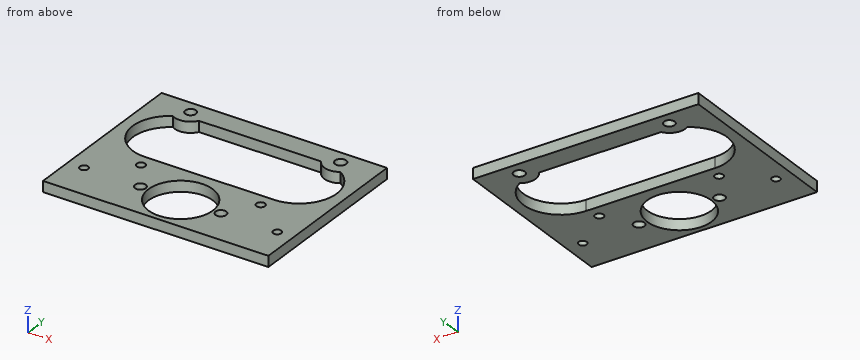
```python
from build123d import *

# Parameters (mm, degrees)
SKETCH1_W           = 133.35
SKETCH1_H           = 104.775
SKETCH1_R           = 2.413
SKETCH1_R_2         = 2.5273
SKETCH1_R_3         = 3.175
SKETCH1_R_4         = 19.05
SKETCH1_R_5         = 3.302
BOSS_EXTRUDE1_DEPTH = 6.35


with BuildPart() as part:
    # Sketch1 → Boss-Extrude1 (new body)
    with BuildSketch(Plane.XY):
        with Locations((0, 30.353)):
            Rectangle(SKETCH1_W, SKETCH1_H)
        with Locations((-57.15, 0)):
            Circle(SKETCH1_R, mode=Mode.SUBTRACT)
        with Locations((-35.41150672, 17.8308)):
            Circle(SKETCH1_R_2, mode=Mode.SUBTRACT)
        with Locations((-23.8125, 0)):
            Circle(SKETCH1_R_3, mode=Mode.SUBTRACT)
        Circle(SKETCH1_R_4, mode=Mode.SUBTRACT)
        with Locations((23.8125, 0)):
            Circle(SKETCH1_R_3, mode=Mode.SUBTRACT)
        with Locations((35.41150672, 17.8308)):
            Circle(SKETCH1_R_2, mode=Mode.SUBTRACT)
        with Locations((57.15, 0)):
            Circle(SKETCH1_R, mode=Mode.SUBTRACT)
        with Locations((44.64152658, 74.693330266)):
            Circle(SKETCH1_R_5, mode=Mode.SUBTRACT)
        with Locations((-44.258181609, 74.921110792)):
            Circle(SKETCH1_R_3, mode=Mode.SUBTRACT)
        with BuildLine():
            Line((-36.078617849, 70.0405), (36.185033541, 70.0405))
            ThreePointArc((36.185033541, 70.0405), (42.31521137, 65.325867347), (49.938818951, 66.624885711))
            ThreePointArc((49.938818951, 66.624885711), (59.454030327, 41.654654783), (38.1, 25.5905))
            Line((38.1, 25.5905), (-38.1, 25.5905))
            ThreePointArc((-38.1, 25.5905), (-59.533112769, 41.9356784), (-49.440641566, 66.929381706))
            ThreePointArc((-49.440641566, 66.929381706), (-42.098222799, 65.644246939), (-36.078617849, 70.0405))
        make_face(mode=Mode.SUBTRACT)
    extrude(amount=-BOSS_EXTRUDE1_DEPTH)


solid = part.part
```
Verification items for the finished model (mm, model axes). Coordinates: 2 decimals unless noted, no trailing zeros. Loops run counter-clockwise (first coordinate to the right, second up) from the corner with the lowest first, then second, coordinate; pieces in that order, holes last. Notation, with made-up numbers: (21, 15) -> (54, 15) arc R14 cw to (54, 31) -> close; hole circle Ø4 at (-11.5, 83). An arc over 180 degrees is marked (long way). Answer in a Markdown table with one row per item.
1) Depth check by flat-ended pin: P1, Ø1, axis at x = -34.5, y = 17, coming from the +Z side; P2, Ø6.5, axis at x = -57.15, y = 0, coming from the -Z side. Enter the tip coordinate at first touch or a pass-through.
The answers:
| item | result |
|---|---|
| P1 | passes through |
| P2 | stops at z = -6.35 |
2) Scan lines: line 1 along Y through (x, z) = (-35, -0.5); line 2 along X through (y, z) = (47.5, -3.25) (3 decimals); line 3 along Y through (x, z) = (43, -3). Record each from-to range of solid material in increasing order. Write a range as from..to.
The answers:
| item | result |
|---|---|
| line 1 | y = -22.03..15.34, 20.32..25.59, 70.04..82.74 |
| line 2 | x = -66.675..-60.323, 60.323..66.675 |
| line 3 | y = -22.03..26.14, 65.18..71.83, 77.56..82.74 |
3) Section check B-B (z = -5.25). Give the number of separate pieces and of enclosed holes in the cut face, and give its area (3 significant figures).
The answers:
| item | result |
|---|---|
| separate pieces | 1 |
| enclosed holes | 10 |
| area | 7,760 mm2 |
4) Section check A-A (x = 0). Record the cut outline in (y, z).
The answers:
| item | result |
|---|---|
| outline | (-22.03, -6.35) -> (-19.05, -6.35) -> (-19.05, 0) -> (-22.03, 0) -> close; (19.05, -6.35) -> (25.59, -6.35) -> (25.59, 0) -> (19.05, 0) -> close; (70.04, -6.35) -> (82.74, -6.35) -> (82.74, 0) -> (70.04, 0) -> close |
5) Section check C-C (y = 6). Record the cut outline in (x, z) (3 decimals).
The answers:
| item | result |
|---|---|
| outline | (-66.675, -6.35) -> (-18.08, -6.35) -> (-18.08, 0) -> (-66.675, 0) -> close; (18.08, -6.35) -> (66.675, -6.35) -> (66.675, 0) -> (18.08, 0) -> close |
6) Section check D-D (x = -51.5). Record the cut outline in (y, z), and give its area (3 significant figures).
The answers:
| item | result |
|---|---|
| outline | (-22.03, -6.35) -> (30.08, -6.35) -> (30.08, 0) -> (-22.03, 0) -> close; (65.55, -6.35) -> (82.74, -6.35) -> (82.74, 0) -> (65.55, 0) -> close |
| area | 440 mm2 |
